Check sheet for the modelled part. Datum: model origin and axes. Units: mm. A direction names the side the tool comes from. Give positions to 0.01 mm unless a question says otherwise; leave off trailing zeros. Order: outer loops, then holes, each group sorted by start corner. A loop starts at its lowest first (then second) coordinate and runs counter-clockwise, first axis right, second up. Notation, with made-up numbers: (65.5, 66) -> (83.5, 66) arc R12 cw to (83.5, 70) -> close; hole circle Ø2 at (11.5, 37). An arc over 180 degrees is marked (long way). Answer in a Markdown table with one row per item. Add a question column.
(1) Release check for a two-part mould opening along X. For faces 1 (the face through (16, -4.826, 20)), 2 (the face through (11, -11, 40.234)), 3 (the face through (31.28, 23.42, 7.78)) record: released by +X, released by -X, zero draft, split by the parting line, or undercut.
(2) Go/stop test with flat-tipped pins: pin 1 (4 mm diameter, centred on y = -17.5, z = 23.5, fed in from +X); pin 2 (2 mm diameter, centred on y = -0.5, z = 6.5, fed in from -X) (3 decimals); pin 3 (5 mm diameter, centred on x = 13.5, z = 18, fed in from +Y). Record where each tip stops, or that it passes through.
(3) Cross-section at C-C (z = 38.5). Record the cut outline in (x, y) (1 decimal), then the cut area to 3 significant figures.
(4) Cross-section at B-B (y = -7). State how many separate pieces and enclosed holes the cut face has, then the cut area to 3 significant figures.
(5) Thickness scan on L1, parallel to X at y = 0, z = 30.5 (1 decimal); L2, parallel to X at y = -6, z = 14; L3, parallel to Y at x = 0, z = 17.5 (1 decimal). Record the ranges inside material, lowest first. Write a range as [from, to].
(6) Set-up check for faces 4 (the face through (30.556, -23.548, 7.776)), 5 (the face through (16, 4.826, 20)): record each of +Z, -Z, +X, -X, +Y, -Y from which the full face is reachable in a straight line by a thin tool's end or side.
```python
from build123d import *

# Parameters (mm, degrees)
F0_R     = 10.16
F1_DEPTH = 15.7734
F2_DEPTH = 40.2336
F3_R     = 3.302


with BuildPart() as f1:
    # F0 (on Top) → F1 (new body)
    with BuildSketch(Plane.XY):
        with BuildLine():
            ThreePointArc((5.046973, -28.125766), (21.917435, -18.334576), (28.575, 0))
            ThreePointArc((28.575, 0), (21.917435, 18.334576), (5.046973, 28.125766))
            ThreePointArc((5.046973, 28.125766), (-28.575, 0), (5.046973, -28.125766))
        make_face()
        with BuildLine():
            ThreePointArc((13.447765, -4.826), (-14.2875, 0), (13.447765, 4.826))
            Line((13.447765, 4.826), (18.5293, 4.826))
            Line((18.5293, 4.826), (18.5293, -4.826))
            Line((18.5293, -4.826), (13.447765, -4.826))
        make_face(mode=Mode.SUBTRACT)
        with BuildLine():
            ThreePointArc((5.046973, 28.125766), (21.917435, 18.334576), (28.575, 0))
            ThreePointArc((28.575, 0), (21.917435, -18.334576), (5.046973, -28.125766))
            Line((5.046973, -28.125766), (56.789061, -18.841007))
            ThreePointArc((56.789061, -18.841007), (34.925, 0), (56.789061, 18.841007))
            Line((56.789061, 18.841007), (5.046973, 28.125766))
        make_face()
        with BuildLine():
            Line((57.88735, 18.643927), (56.789061, 18.841007))
            ThreePointArc((56.789061, 18.841007), (34.925, 0), (56.789061, -18.841007))
            Line((56.789061, -18.841007), (57.88735, -18.643927))
            ThreePointArc((57.88735, -18.643927), (68.764063, -12.007752), (73.025, 0))
            ThreePointArc((73.025, 0), (68.764063, 12.007752), (57.88735, 18.643927))
        make_face()
        with Locations((53.975, 0)):
            Circle(F0_R, mode=Mode.SUBTRACT)
        with BuildLine():
            ThreePointArc((57.88735, 18.643927), (57.339649, 18.75051), (56.789061, 18.841007))
            Line((56.789061, 18.841007), (57.88735, 18.643927))
        make_face()
        with BuildLine():
            Line((57.88735, -18.643927), (56.789061, -18.841007))
            ThreePointArc((56.789061, -18.841007), (57.339649, -18.75051), (57.88735, -18.643927))
        make_face()
    extrude(amount=F1_DEPTH)

    # F0 (on Top) → F2 (join)
    with BuildSketch(Plane.XY):
        with BuildLine():
            ThreePointArc((5.046973, -28.125766), (21.917435, -18.334576), (28.575, 0))
            ThreePointArc((28.575, 0), (21.917435, 18.334576), (5.046973, 28.125766))
            ThreePointArc((5.046973, 28.125766), (-28.575, 0), (5.046973, -28.125766))
        make_face()
        with BuildLine():
            ThreePointArc((13.447765, -4.826), (-14.2875, 0), (13.447765, 4.826))
            Line((13.447765, 4.826), (18.5293, 4.826))
            Line((18.5293, 4.826), (18.5293, -4.826))
            Line((18.5293, -4.826), (13.447765, -4.826))
        make_face(mode=Mode.SUBTRACT)
    extrude(amount=F2_DEPTH)

    # F3
    f3_edges = [f1.edges().sort_by_distance(p)[0] for p in [
        (-5.046973, 28.125766, 40.2336),
    ]]
    fillet(f3_edges, radius=F3_R)


solid = f1.part
```
Answer below:
| question | item | result |
|---|---|---|
| 1 | face 1 | undercut |
| 1 | face 2 | zero draft |
| 1 | face 3 | released by +X |
| 2 | pin 1 | stops at x = 24.01 |
| 2 | pin 2 | stops at x = -28.575 |
| 2 | pin 3 | stops at y = 26.81 |
| 3 | outline | circle Ø56.4 at (0, 0); hole (13.4, -4.8) -> (18.5, -4.8) -> (18.5, 4.8) -> (13.4, 4.8) arc R14.3 ccw (long way) to start |
| 3 | area | 1,810 mm² |
| 4 | separate pieces | 3 |
| 4 | enclosed holes | 0 |
| 4 | area | 1,680 mm² |
| 5 | L1 | x = [-28.6, -14.3], [18.5, 28.6] |
| 5 | L2 | x = [-27.94, -12.97], [12.97, 45.78], [62.17, 72.06] |
| 5 | L3 | y = [-28.6, -14.3], [14.3, 28.6] |
| 6 | face 4 | +Z, -Z, +X, -Y |
| 6 | face 5 | +Z, -Z |
